from build123d import *

# Parameters (mm, degrees)
F0_W     = 76.2
F0_H     = 127
F0_R     = 5.715
F0_W_2   = 38.1
F0_H_2   = 6.35
F1_DEPTH = 6.35


with BuildPart() as f1:
    # F0 (on Front) → F1 (new body)
    with BuildSketch(Plane.XZ):
        Rectangle(F0_W, F0_H)
        with Locations((0, -53.34)):
            Circle(F0_R, mode=Mode.SUBTRACT)
        with Locations((0, 22.225)):
            Rectangle(F0_W_2, F0_H_2, mode=Mode.SUBTRACT)
    extrude(amount=F1_DEPTH)


solid = f1.part
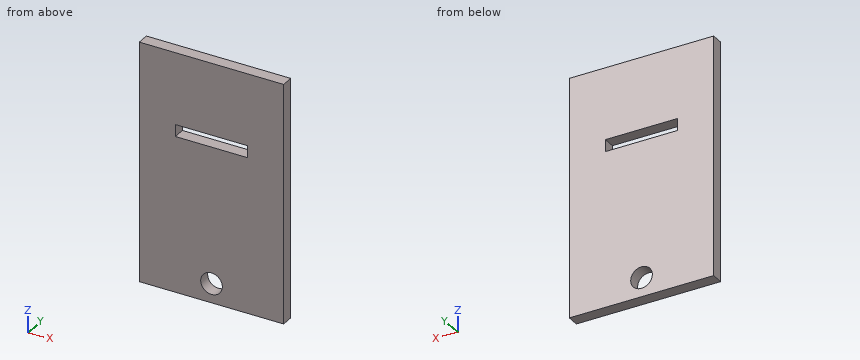
Build history of the part. All positions in model axes, mm. Round coordinates to 2 decimals unless told otherwise and drop trailing zeros. Write each loop counter-clockwise with the first axis right and the second up, starting at its lowest first coordinate (ties: lowest second). Pieces come first, ordered by that corner, then holes. Notation, with made-up numbers: (11.25, 3) -> (22.25, 3) arc R19 cw to (22.25, 9) -> close; hole circle Ø8 at (8, 12.5). An arc over 180 degrees is marked (long way). Write item = value, one per line.
(1) Probe L1, parallel to Z at x = 0, y = -4.75 (3 decimals); L2, parallel to Z at x = 6, y = -4.5; L3, parallel to X at y = -2, z = -49.5. List the from-to ranges inside material, lowest first.
Answer:
L1 = -63.5 to -59.055, -47.625 to 19.05, 25.4 to 63.5
L2 = -63.5 to 19.05, 25.4 to 63.5
L3 = -38.1 to -4.23, 4.23 to 38.1
(2) Band-saw the part on D-D (x = 12.5). Give the cut face in (y, z), then the cut area to 3 significant figures.
Answer:
outline = (-6.35, -63.5) -> (0, -63.5) -> (0, 19.05) -> (-6.35, 19.05) -> close; (-6.35, 25.4) -> (0, 25.4) -> (0, 63.5) -> (-6.35, 63.5) -> close
area = 766 mm2
(3) Band-saw the part on A-A (x = 0). Give the cut face in (y, z) (3 decimals), then the cut area to 3 significant figures.
Answer:
outline = (-6.35, -63.5) -> (0, -63.5) -> (0, -59.055) -> (-6.35, -59.055) -> close; (-6.35, -47.625) -> (0, -47.625) -> (0, 19.05) -> (-6.35, 19.05) -> close; (-6.35, 25.4) -> (0, 25.4) -> (0, 63.5) -> (-6.35, 63.5) -> close
area = 694 mm2
(4) Band-saw the part on B-B (z = -53.34). Give the cut face in (x, y) (3 decimals).
Answer:
outline = (-38.1, -6.35) -> (-5.715, -6.35) -> (-5.715, 0) -> (-38.1, 0) -> close; (5.715, -6.35) -> (38.1, -6.35) -> (38.1, 0) -> (5.715, 0) -> close
(5) Band-saw the part on C-C (y = -3.25). Give the cut face in (x, z) (3 decimals), then the cut area to 3 significant figures.
Answer:
outline = (-38.1, -63.5) -> (38.1, -63.5) -> (38.1, 63.5) -> (-38.1, 63.5) -> close; hole (-19.05, 19.05) -> (19.05, 19.05) -> (19.05, 25.4) -> (-19.05, 25.4) -> close; hole circle Ø11.43 at (0, -53.34)
area = 9,330 mm2
